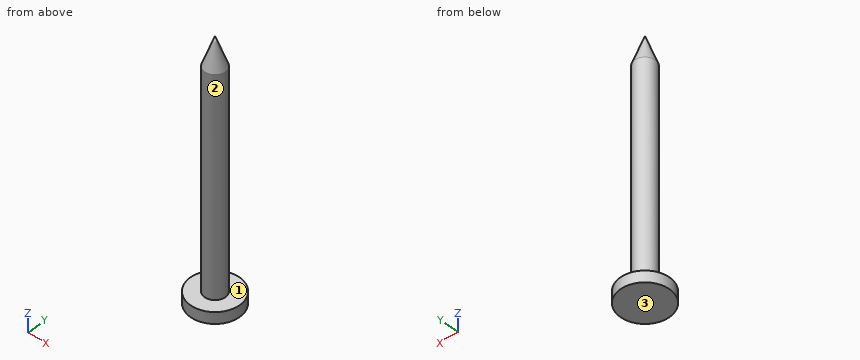
from build123d import *

# Parameters (mm, degrees)
F0_R      = 3.25
F0_R_2    = 1.375
F1_DEPTH  = 1.5
F2_DEPTH  = 30
F2_FACE_R = 1.375
F3_DEPTH  = 5
F3_TAPER  = 20


with BuildPart() as f1:
    # F0 (on Top) → F1 (new body)
    with BuildSketch(Plane.XY):
        Circle(F0_R)
        Circle(F0_R_2, mode=Mode.SUBTRACT)
    extrude(amount=F1_DEPTH)

    # F0 (on Top) → F2 (join)
    with BuildSketch(Plane.XY):
        Circle(F0_R_2)
    extrude(amount=F2_DEPTH)

    # F2_face (on face) → F3 (join)
    with BuildSketch(Plane.XY.offset(30)):
        Circle(F2_FACE_R)
    extrude(amount=F3_DEPTH, taper=F3_TAPER)


solid = f1.part
Check sheet for the modelled part. Datum: model origin and axes. Units: mm. Face numbers are marked on the shaded views. Round coordinates to 2 decimals unless told otherwise and drop trailing zeros. Loops run counter-clockwise (first coordinate to the right, second up) from the corner with the lowest first, then second, coordinate; pieces in that order, holes last. Notation, with made-up numbers: M -2,18.5 L 12,18.5 A23 ccw 12,43.5 Z; hole C 7,57 d1. An arc over 180 degrees is marked long. One line per item, written item: value.
(1) Sectioned sample at A-A, the plane x = -2.25. Record the cut outline in (y, z).
Computed values:
outline: M -2.35,0 L 2.35,0 L 2.35,1.5 L -2.35,1.5 Z
(2) Depth check by flat-ended pin: pin 1 Ø3 at (x, z) = (0, 30) entering from +Y (3 decimals); pin 2 Ø2 at (x, z) = (1, 22.5) entering from -Y (3 decimals). Enter the tip coordinate at first touch or a pass-through.
Computed values:
pin 1: stops at y = 1.375
pin 2: stops at y = -1.375
(3) Release check for a two-part mould opening along Z. For the marked faces 1, 2 and 3 record: +Z half, -Z half, draft (parallel to the pull), parting line (faces both ways), or undercut.
Computed values:
face 1: +Z half
face 2: draft
face 3: -Z half
(4) Sectioned sample at C-C, the plane y = 2.75. Record the cut outline in (x, z), then the cut area to 3 significant figures.
Computed values:
outline: M -1.73,0 L 1.73,0 L 1.73,1.5 L -1.73,1.5 Z
area: 5.20 mm^2
(5) Sectioned sample at B-B, the plane z = 19.5. Record the cut outline in (x, y) (3 decimals), then the cut area to 3 significant figures.
Computed values:
outline: C 0,0 d2.75
area: 5.94 mm^2
(6) Thickness scan on line 1 (Z direction, x = -2, y = 1); line 2 (X direction, y = 0.75, z = 13); line 3 (X direction, y = -1, z = 21). Record the ranges inside material, lowest first.
Computed values:
line 1: z = 0 to 1.5
line 2: x = -1.15 to 1.15
line 3: x = -0.94 to 0.94
